Build history of the part. All positions in model axes, mm. Face numbers are marked on the shaded views. A direction names the side the tool comes from. Give positions to 0.01 mm unless a question says otherwise; leave off trailing zeros. Order: outer loops, then holes, each group sorted by start corner. A loop starts at its lowest first (then second) coordinate and runs counter-clockwise, first axis right, second up. Notation, with made-up numbers: M -0.75,11.25 L 54.25,11.25 A16 cw 54.25,15.25 Z; hole C 24,43.5 d1. An arc over 180 degrees is marked long. Use CSV: the item, a comma, the result in double quotes. Start each with the question number.
Item 1: Two-plate mould, pull along X, no slides. Class the marked faces 4, 5 and 6: pulls with the +X half, pulls with the -X half, needs draft (parallel to the pull), parting line crosses it, or undercut.
Item 2: Band-saw the part on C-C on x = 25. Write the cut outline in (y, z), plus the area to 3 significant figures.
Item 3: Wall check: line 1 along Y through (x, z) = (8, 33); line 2 along Y through (x, z) = (16.5, -31); line 3 along Y through (x, z) = (37, 28). Give the ranges that are in metal, low to high.
Item 4: Pin check, flat tips, straight feed: P1, Ø6, axis at x = 14, y = 53, coming from the -Z side; P2, Ø11, axis at y = 46.5, z = 25, coming from the +X side; P3, Ø8, axis at x = 30, y = 30.5, coming from the +Z side; P4, Ø9, axis at y = 11.25, z = 33, coming from the -X side. Stop position of each tip, or through.
Item 5: Which spindle directions (+Z, -Z, +X, -X, +Y, -Y) get a long thin tool onto all of the face, cutting with end or side? Do the marked faces 1, 2 and 3. Say none if no direction does.
Item 6: Band-saw the part on B-B on z = 33. Write the cut outline in (x, y).
Item 7: Band-saw the part on A-A on y = 11.25. Write the cut outline in (x, z).
Item 8: Band-saw the part on D-D on z = -3. Write the cut outline in (x, y), plus the area to 3 significant figures.
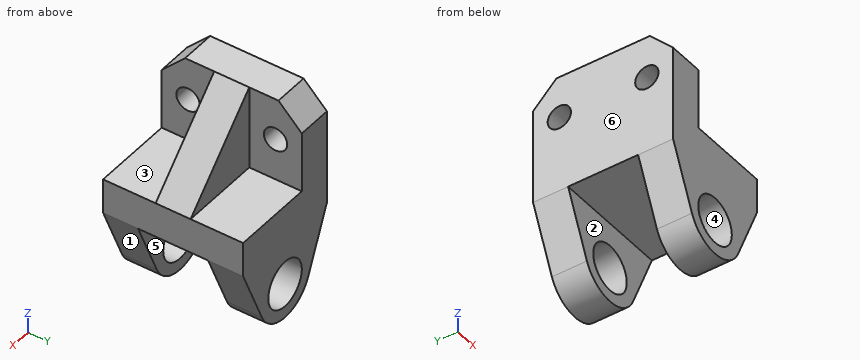
Autodesk Inventor part; units mm, degrees
ref_plane "Work Plane1" through (0, 30, 15) normal (0, 1, 0) x (1, 0, 0)
ref_plane "Work Plane3" through (15, 22.5, 51) normal (0, -1, 0) x (0, 0, -1)
ref_plane "YZ Plane" through (0, 0, 0) normal (1, 0, 0) x (0, 1, 0)
sketch "Sketch1" plane through (0, 0, 0) normal (0, 0, 1) x (1, 0, 0)
  line L0 (0, 60) -> (50, 60)
  line L1 (50, 60) -> (50, 0)
  line L2 (50, 0) -> (0, 0)
  line L3 (0, 0) -> (0, 60)
  dimension "d0" = 50
  dimension "d1" = 60
extrude "Extrusion1" add sketch "Sketch1" along normal blind 15
sketch "Sketch2" plane through (0, 60, 0) normal (0, 1, 0) x (1, 0, 0)
  circle A0 centre (25, 20) radius 10
  circle A1 centre (25, 20) radius 15
  line L0 (50, 0) -> (0, 0)
  line L1 (25, 0) -> (25, 35.9147) construction
  line L2 (0, 0) -> (0, -15) construction
  line L3 (0, 0) -> (11.2339, 25.9577)
  line L4 (50, 0) -> (50, -15)
  line L5 (50, 0) -> (38.7661, 25.9577)
  dimension "d4" = 20
  dimension "d5" = 30
  dimension "d6" = 20
extrude "Extrusion2" add sketch "Sketch2" against normal blind 15
ref_plane "Work Plane1" through (0, 30, 15) normal (0, 1, 0) x (1, 0, 0)
mirror "Mirror1" about plane through (0, 30, 15) normal (0, 1, 0) of "Extrusion2"
sketch "Sketch3" plane through (0, 0, 15) normal (0, 0, 1) x (1, 0, 0)
  line L0 (50, 0) -> (50, 60)
  line L1 (0, 60) -> (0, 0)
  line L2 (50, 60) -> (0, 60)
  line L3 (0, 0) -> (15, 0)
  line L4 (15, 0) -> (15, 60)
  line L5 (15, 60) -> (0, 60)
  line L6 (0, 60) -> (0, 0)
  dimension "d12" = 15
extrude "Extrusion3" add sketch "Sketch3" along normal blind 36
ref_plane "Work Plane3" through (15, 22.5, 51) normal (0, -1, 0) x (0, 0, -1)
sketch "Sketch5" plane through (15, 22.5, 51) normal (0, -1, 0) x (0, 0, -1)
  line L0 (36, 0) -> (0, 0)
  line L1 (0, 0) -> (36, 35)
  line L2 (36, 0) -> (36, 35)
  point P0 (51, -15)
extrude "Extrusion4" add sketch "Sketch5" against normal blind 15
chamfer "Chamfer1" distance 10 angle 45 2 edges at (7.5, 0, 51) (7.5, 60, 51)
sketch "Sketch7" plane through (15, 37.5, 15) normal (1, 0, 0) x (0, 0, -1)
  line L0 (0, 22.5) -> (-26, 22.5)
  line L1 (-36, 0) -> (0, 0)
  line L2 (0, 0) -> (0, 22.5)
  line L3 (-36, 0) -> (-36, 12.5)
  line L4 (-5.5947, -7.5) -> (-36, -7.5) construction
  line L5 (-36, 12.5) -> (-36, -27.5) construction
  point P0 (15, -37.5)
  point P1 (-18, 11.25)
  point P2 (-18, -26.25)
  dimension "d28" = 11.25
  dimension "d29" = 22.5
  dimension "d30" = 36
  dimension "d31" = 18
hole "Hole2" at (15, 48.75, 33) at (15, 11.25, 33) direction (-1, 0, 0) diameter 10 end through all
properties part number "01"
Model answer:
1,face 4,"undercut"
1,face 5,"needs draft"
1,face 6,"pulls with the -X half"
2,outline,"M 0,-35 L 15,-35 L 15,-30 L 0,-30 Z; M 0,-10 L 15,-10 L 15,0 L 45,0 L 45,-10 L 60,-10 L 60,15 L 37.5,15 L 37.5,40.71 L 22.5,40.71 L 22.5,15 L 0,15 Z; M 45,-35 L 60,-35 L 60,-30 L 45,-30 Z"
2,area,"1,740 mm^2"
3,line 1,"y = 0 to 6.25, 16.25 to 43.75, 53.75 to 60"
3,line 2,"y = 0 to 15, 45 to 60"
3,line 3,"y = 22.5 to 37.5"
4,P1,"stops at z = -32.69"
4,P2,"stops at x = 15"
4,P3,"stops at z = 39.69"
4,P4,"passes through"
5,face 1,"-Z, +X, +Y, -Y"
5,face 2,"-Z, +X, -X"
5,face 3,"+Z, +X, -Y"
6,outline,"M 0,0 L 15,0 L 15,6.25 L 0,6.25 Z; M 0,16.25 L 15,16.25 L 15,22.5 L 32.5,22.5 L 32.5,37.5 L 15,37.5 L 15,43.75 L 0,43.75 Z; M 0,53.75 L 15,53.75 L 15,60 L 0,60 Z"
7,outline,"M 0,0 L 11.23,-25.96 A15 ccw 38.77,-25.96 L 50,0 L 50,15 L 15,15 L 15,28 L 0,28 Z; M 0,38 L 15,38 L 15,51 L 0,51 Z; hole C 25,-20 d20"
8,outline,"M 1.3,0 L 48.7,0 L 48.7,15 L 1.3,15 Z; M 1.3,45 L 48.7,45 L 48.7,60 L 1.3,60 Z"
8,area,"1,420 mm^2"
